CAD build for the part. Positions are in the model's coordinates, mm. A direction names the side the tool comes from. Coordinates: 2 decimals unless noted, no trailing zeros. Loops run counter-clockwise (first coordinate to the right, second up) from the corner with the lowest first, then second, coordinate; pieces in that order, holes last. Notation, with made-up numbers: (66.25, 14) -> (105.25, 14) arc R13 ccw to (105.25, 19) -> close; hole circle Ø7 at (34.25, 74.25). An arc over 180 degrees is marked (long way). Write item = value, one per line. Start each with the question number.
(1) Drill centre lines: line 1 (Y direction, x = 9, z = -10); line 2 (Z direction, x = 10.25, y = 0.55); line 3 (Z direction, x = 5, y = 0.4). Where is each one in solid material? Low to high. Write a range as from..to.
(2) Band-saw the part on D-D (z = -10). Write the cut outline in (x, y), and give its area (3 significant figures).
(3) Tool access for faces 1 (the face through (12.3, 0.5, -1.884)), 2 (the face through (6.3, 0.5, -0.933)), 3 (the face through (1, 1.2, -5)): list every direction of +Z, -Z, +X, -X, +Y, -Y with a clear straight run to the whole face (end or side of a thin tool).
(4) Band-saw the part on C-C (z = -5.5). Write the cut outline in (x, y), and give its area (3 significant figures).
(5) Flat gauge pin, fed straight in: P1, Ø2, axis at x = 10.5, z = -5.5, coming from the +Y side. Where does the tip first touch, or does it go through?
(6) Band-saw the part on B-B (x = 10). Write the cut outline in (y, z), and give its area (3 significant figures).
(7) Band-saw the part on A-A (y = 0.6). Write the cut outline in (x, z).
```python
from build123d import *

# Parameters (mm, degrees)
SKETCH1_W           = 15
SKETCH1_H           = 11
BOSS_EXTRUDE1_DEPTH = 1
CUT_EXTRUDE3_DEPTH  = 19.62793601
CUT_EXTRUDE4_DEPTH  = 19.62793601
FILLET3_R           = 0.25
FILLET4_R           = 0.25
SKETCH8_R           = 7.705
BOSS_EXTRUDE2_DEPTH = 0.2
SKETCH12_W          = 14.564245133
SKETCH12_H          = 17.019207238
CUT_EXTRUDE5_DEPTH  = 21.020290333
FILLET5_R           = 0.25


with BuildPart() as part:
    # Sketch1 → Boss-Extrude1 (new body)
    with BuildSketch(Plane(origin=(0, 0, 0), x_dir=(1, 0, 0), z_dir=(0, 1, 0))):
        with Locations((7.5, 5.5)):
            Rectangle(SKETCH1_W, SKETCH1_H)
    extrude(amount=BOSS_EXTRUDE1_DEPTH)

    # Sketch4 → Cut-Extrude3 (cut, through all)
    with BuildSketch(Plane(origin=(0, 1, 0), x_dir=(1, 0, 0), z_dir=(0, 1, 0))):
        Polygon((4.749438202, 0), (5.682709114, 0.933270911), (7.024594257, 0.933270911), (7.024594257, 0), align=None)
    extrude(amount=-CUT_EXTRUDE3_DEPTH, mode=Mode.SUBTRACT)

    # Sketch6 → Cut-Extrude4 (cut, through all)
    with BuildSketch(Plane(origin=(0, 1, 0), x_dir=(1, 0, 0), z_dir=(0, 1, 0))):
        Polygon((8.909238452, 0), (9.826092385, 1.883520599), (15, 1.883520599), (15, 0), align=None)
    extrude(amount=-CUT_EXTRUDE4_DEPTH, mode=Mode.SUBTRACT)

    # Fillet3
    fillet3_edges = [part.edges().sort_by_distance(p)[0] for p in [
        (15, 0.5, -1.883520599),
    ]]
    fillet(fillet3_edges, radius=FILLET3_R)

    # Fillet4
    fillet4_edges = [part.edges().sort_by_distance(p)[0] for p in [
        (7.024594257, 0.5, 0),
    ]]
    fillet(fillet4_edges, radius=FILLET4_R)

    # Sketch8 → Boss-Extrude2 (add)
    with BuildSketch(Plane(origin=(0, 1, 0), x_dir=(1, 0, 0), z_dir=(0, 1, 0))):
        with Locations(Location((-5.396795531, 5.5, 0), (0, 0, 45.538670416))):
            Circle(SKETCH8_R)
    extrude(amount=BOSS_EXTRUDE2_DEPTH)

    # Sketch12 → Cut-Extrude5 (cut, through all)
    with BuildSketch(Plane(origin=(0, 1.2, 0), x_dir=(1, 0, 0), z_dir=(0, 1, 0))):
        with Locations((-7.282122567, 5.49450546)):
            Rectangle(SKETCH12_W, SKETCH12_H)
    extrude(amount=-CUT_EXTRUDE5_DEPTH, mode=Mode.SUBTRACT)

    # Fillet5
    fillet5_edges = [part.edges().sort_by_distance(p)[0] for p in [
        (15, 0.5, -11),
        (0, 0.5, 0),
        (0, 0.5, -11),
    ]]
    fillet(fillet5_edges, radius=FILLET5_R)


solid = part.part
```
Findings below:
q1.line_1 = 0..1
q1.line_2 = -11..-1.88
q1.line_3 = -11..-0.25
q2.outline = (0, 0) -> (15, 0) -> (15, 1) -> (0.86, 1) -> (0.86, 1.2) -> (0, 1.2) -> close
q2.area = 15.2 mm²
q3.face_1 = +Z, +X, +Y, -Y
q3.face_2 = +Z, +Y, -Y
q3.face_3 = +Z, -Z, +X, -X, +Y
q4.outline = (0, 0) -> (15, 0) -> (15, 1) -> (2.31, 1) -> (2.31, 1.2) -> (0, 1.2) -> close
q4.area = 15.5 mm²
q5.P1 = 1
q6.outline = (0, -11) -> (1, -11) -> (1, -1.88) -> (0, -1.88) -> close
q6.area = 9.12 mm²
q7.outline = (0, -10.75) arc R0.25 ccw to (0.25, -11) -> (14.75, -11) arc R0.25 ccw to (15, -10.75) -> (15, -2.13) arc R0.25 ccw to (14.75, -1.88) -> (9.83, -1.88) -> (8.91, 0) -> (7.27, 0) arc R0.25 ccw to (7.02, -0.25) -> (7.02, -0.93) -> (5.68, -0.93) -> (4.75, 0) -> (0.25, 0) arc R0.25 ccw to (0, -0.25) -> close
